from build123d import *

# Parameters (mm, degrees)
SKETCH2_W           = 10.16
SKETCH2_H           = 76.2
SKETCH2_W_2         = 50
SKETCH2_H_2         = 10.16
SKETCH2_H_3         = 89.916
SKETCH2_R           = 3.175
SKETCH2_H_4         = 10
SKETCH2_R_2         = 4.7625
BOSS_EXTRUDE1_DEPTH = 10.16
SKETCH6_W           = 14
SKETCH6_H           = 112.399749
CUT_EXTRUDE1_DEPTH  = 15.24
CUT_EXTRUDE2_START  = -10.16
SKETCH11_R          = 4
CUT_EXTRUDE2_DEPTH  = 10.16


with BuildPart() as part:
    # Sketch2 → Boss-Extrude1 (new body)
    with BuildSketch(Plane.XY):
        with BuildLine():
            Line((-408.300796745, 142.616356263), (-408.921789204, 152.75736057))
            Line((-408.921789204, 152.75736057), (-459.721789204, 152.75736057))
            Line((-459.721789204, 152.75736057), (-459.721789204, 76.39736057))
            Line((-459.721789204, 76.39736057), (-469.435656714, 76.39736057))
            Line((-469.435656714, 76.39736057), (-469.435656714, 25.59736057))
            Line((-469.435656714, 25.59736057), (-459.721789204, 25.59736057))
            Line((-459.721789204, 25.59736057), (-459.721789204, -230.782639429))
            ThreePointArc((-459.721789204, -230.782639429), (-437.403325931, -284.664176156), (-383.521789204, -306.982639429))
            Line((-383.521789204, -306.982639429), (-303.52, -306.982639429))
            Line((-303.52, -306.982639429), (-270.8, -306.98263943))
            Line((-270.8, -306.98263943), (-270.8, -317.14263943))
            Line((-270.8, -317.14263943), (-220, -317.14263943))
            Line((-220, -317.14263943), (-220, -306.98263943))
            Line((-220, -306.98263943), (-55.8292, -306.982639429))
            Line((-55.8292, -306.982639429), (-55.8292, -317.14263943))
            Line((-55.8292, -317.14263943), (55.8292, -317.14263943))
            Line((55.8292, -317.14263943), (55.8292, -306.982639429))
            Line((55.8292, -306.982639429), (220, -306.98263943))
            Line((220, -306.98263943), (220, -317.14263943))
            Line((220, -317.14263943), (270.8, -317.14263943))
            Line((270.8, -317.14263943), (270.8, -306.98263943))
            Line((270.8, -306.98263943), (303.52, -306.982639429))
            Line((303.52, -306.982639429), (383.521789204, -306.982639429))
            ThreePointArc((383.521789204, -306.982639429), (437.403325931, -284.664176156), (459.721789204, -230.782639429))
            Line((459.721789204, -230.782639429), (459.721789204, 25.59736057))
            Line((459.721789204, 25.59736057), (469.435656714, 25.59736057))
            Line((469.435656714, 25.59736057), (469.435656714, 76.39736057))
            Line((469.435656714, 76.39736057), (459.721789204, 76.39736057))
            Line((459.721789204, 76.39736057), (459.721789204, 152.75736057))
            Line((459.721789204, 152.75736057), (408.921789204, 152.75736057))
            Line((408.921789204, 152.75736057), (408.921789204, 142.616356263))
            Line((408.921789204, 142.616356263), (332.721789204, 142.616356263))
            Line((332.721789204, 142.616356263), (332.721789204, 152.75736057))
            Line((332.721789204, 152.75736057), (84.450547773, 152.75736057))
            Line((84.450547773, 152.75736057), (84.450547773, 316.728644457))
            Line((84.450547773, 316.728644457), (-84.450547773, 316.728644457))
            Line((-84.450547773, 316.728644457), (-84.450547773, 152.75736057))
            Line((-84.450547773, 152.75736057), (-332.100796745, 152.75736057))
            Line((-332.100796745, 152.75736057), (-332.100796745, 142.616356263))
            Line((-332.100796745, 142.616356263), (-408.300796745, 142.616356263))
        make_face()
        with Locations((-205.08, -256.782661115)):
            Rectangle(SKETCH2_W, SKETCH2_H, mode=Mode.SUBTRACT)
        with Locations((-84.92, -256.782661115)):
            Rectangle(SKETCH2_W, SKETCH2_H, mode=Mode.SUBTRACT)
        with Locations((-345.16, -186.334154613)):
            Rectangle(SKETCH2_W_2, SKETCH2_H_2, mode=Mode.SUBTRACT)
        with Locations((-310.712287657, -172.10863943)):
            Rectangle(SKETCH2_W, SKETCH2_H_3, mode=Mode.SUBTRACT)
        with Locations((-436.123522935, -86.033983844)):
            Circle(SKETCH2_R, mode=Mode.SUBTRACT)
        with Locations((-405.323522935, -86.033983844)):
            Circle(SKETCH2_R, mode=Mode.SUBTRACT)
        with Locations((-235.16, -186.254154613)):
            Rectangle(SKETCH2_W_2, SKETCH2_H_4, mode=Mode.SUBTRACT)
        with Locations((310.712287657, -172.10863943)):
            Rectangle(SKETCH2_W, SKETCH2_H_3, mode=Mode.SUBTRACT)
        with Locations((-345.16, -74.366988355)):
            Rectangle(SKETCH2_W_2, SKETCH2_H_2, mode=Mode.SUBTRACT)
        with Locations((-310.712287657, 7.72336057)):
            Rectangle(SKETCH2_W, SKETCH2_H_3, mode=Mode.SUBTRACT)
        Polygon((-210.16, -79.446988355), (-260.16, -79.446988355), (-260.16, -69.446988355), (-210.16, -69.446988355), (-210.16, -8.96237531), (-200, -8.96237531), (-200, -85.16237531), (-210.16, -85.16237531), align=None, mode=Mode.SUBTRACT)
        with Locations((-84.92, -47.06237531)):
            Rectangle(SKETCH2_W, SKETCH2_H, mode=Mode.SUBTRACT)
        with Locations((-436.123522935, 60.016016156)):
            Circle(SKETCH2_R, mode=Mode.SUBTRACT)
        with Locations((-405.323522935, 60.016016156)):
            Circle(SKETCH2_R, mode=Mode.SUBTRACT)
        with Locations((-420.723522935, 122.038203417)):
            Circle(SKETCH2_R, mode=Mode.SUBTRACT)
        with Locations((-172.2755, 25.75736057)):
            Circle(SKETCH2_R_2, mode=Mode.SUBTRACT)
        with Locations((-81.7245, 25.75736057)):
            Circle(SKETCH2_R_2, mode=Mode.SUBTRACT)
        with Locations((-172.2755, 127.35736057)):
            Circle(SKETCH2_R_2, mode=Mode.SUBTRACT)
        with Locations((-81.7245, 127.35736057)):
            Circle(SKETCH2_R_2, mode=Mode.SUBTRACT)
        with Locations((310.712287657, 7.72336057)):
            Rectangle(SKETCH2_W, SKETCH2_H_3, mode=Mode.SUBTRACT)
        with Locations((81.7245, 25.75736057)):
            Circle(SKETCH2_R_2, mode=Mode.SUBTRACT)
        with Locations((81.7245, 127.35736057)):
            Circle(SKETCH2_R_2, mode=Mode.SUBTRACT)
        with Locations((172.2755, 25.75736057)):
            Circle(SKETCH2_R_2, mode=Mode.SUBTRACT)
        with Locations((172.2755, 127.35736057)):
            Circle(SKETCH2_R_2, mode=Mode.SUBTRACT)
    extrude(amount=-BOSS_EXTRUDE1_DEPTH)

    # Sketch6 → Cut-Extrude1 (cut)
    with BuildSketch(Plane(origin=(0, 0, -10.16), x_dir=(-1, 0, 0), z_dir=(0, 0, -1))):
        with Locations((386.721789204, 30.216607763)):
            Rectangle(SKETCH6_W, SKETCH6_H)
        with Locations((386.721789204, -194.582890237)):
            Rectangle(SKETCH6_W, SKETCH6_H)
    cut_extrude1 = extrude(amount=-CUT_EXTRUDE1_DEPTH, mode=Mode.SUBTRACT)

    # Mirror1: Cut-Extrude1 across plane
    add(cut_extrude1.mirror(Plane(origin=(0, 0, 0), x_dir=(0, 0, 1), z_dir=(1, 0, 0))), mode=Mode.SUBTRACT)

    # Sketch11 → Cut-Extrude2 (cut)
    with BuildSketch(Plane.XY.offset(CUT_EXTRUDE2_START)):
        with Locations((-172.6526, -269.442639029)):
            Circle(SKETCH11_R)
        with BuildLine():
            Line((-168.652969828, -239.497030969), (-176.652230173, -239.497030969))
            ThreePointArc((-176.652230173, -239.497030969), (-172.6526, -243.442639029), (-168.652969828, -239.497030969))
        make_face()
        with BuildLine():
            ThreePointArc((-168.6526, -239.442639029), (-172.679796599, -235.442731487), (-176.652230173, -239.497030969))
            Line((-176.652230173, -239.497030969), (-168.652969828, -239.497030969))
            ThreePointArc((-168.652969828, -239.497030969), (-168.652692458, -239.469835628), (-168.6526, -239.442639029))
        make_face()
        with BuildLine():
            ThreePointArc((-113.3474, -239.442639029), (-117.374596599, -235.442731487), (-121.347030173, -239.497030969))
            Line((-121.347030173, -239.497030969), (-113.347769828, -239.497030969))
            ThreePointArc((-113.347769828, -239.497030969), (-113.347492458, -239.469835628), (-113.3474, -239.442639029))
        make_face()
        with BuildLine():
            Line((-113.347769828, -239.497030969), (-121.347030173, -239.497030969))
            ThreePointArc((-121.347030173, -239.497030969), (-117.3474, -243.442639029), (-113.347769828, -239.497030969))
        make_face()
        with Locations((-117.3474, -269.442639029)):
            Circle(SKETCH11_R)
    extrude(amount=CUT_EXTRUDE2_DEPTH, mode=Mode.SUBTRACT)


solid = part.part
Input: part model. Units: mm. Frame: model coordinates. Coordinates: 2 decimals unless noted, no trailing zeros. Loops run counter-clockwise (first coordinate to the right, second up) from the corner with the lowest first, then second, coordinate; pieces in that order, holes last. Notation, with made-up numbers: (33.5, 30) -> (58.5, 30) arc R27 cw to (58.5, 46) -> close; hole circle Ø1 at (-32, 8.5). An arc over 180 degrees is marked (long way). Write item = value, one per line. Start each with the question number.
Item 1: Cut plane D-D, the plane y = 194. Return loops of the section in (x, z), plus the area to 3 significant figures.
Item 2: Mould query, pull axis Z, two halves, no side actions, for faces 1 (the face through (-7, -66, -10.16)), 2 (the face through (-7, -66, 0)), 3 (the face through (-437.99, -284.07, -5.01)). Classes: pulls with the +Z half, pulls with the -Z half, needs draft (parallel to the pull), parting line crosses it, or undercut.
Item 3: Cut plane C-C, the plane z = -6.75. Count the separate pieces of the cut face and the enclosed holes in it, plus the area to 3 significant figures.
Item 4: First-contact query: P1, Ø3, axis at y = -83.5, z = -4.5, coming from the +X side; P2, Ø3, axis at y = -243.5, z = -3.5, coming from the +X side; P3, Ø3, axis at x = 388.5, z = -3, coming from the -Y side. Flat tips, straight axial feed; report the tip coordinate or a pass-through.
Item 5: Cut plane A-A, the plane x = -343.5. Return loops of the section in (y, z), plus the area to 3 significant figures.
Item 6: Cut plane B-B, the plane x = 127.5. Return loops of the section in (y, z).
Item 7: Material intervals for line 1 (Y direction, x = -172.5, z = -0.75); line 2 (X direction, y = -132.5, z = -8); line 3 (X direction, y = -6, z = -4), sorted ascending.
Ans:
q1.outline = (-84.45, -10.16) -> (84.45, -10.16) -> (84.45, 0) -> (-84.45, 0) -> close
q1.area = 1,720 mm²
q2.face_1 = pulls with the -Z half
q2.face_2 = pulls with the +Z half
q2.face_3 = needs draft
q3.separate_pieces = 1
q3.enclosed_holes = 32
q3.area = 434,000 mm²
q4.P1 = 459.72
q4.P2 = 458.89
q4.P3 = -306.9
q5.outline = (-306.98, -10.16) -> (-191.41, -10.16) -> (-191.41, 0) -> (-306.98, 0) -> close; (-181.25, -10.16) -> (-79.45, -10.16) -> (-79.45, 0) -> (-181.25, 0) -> close; (-69.29, -10.16) -> (142.62, -10.16) -> (142.62, 0) -> (-69.29, 0) -> close
q5.area = 4,360 mm²
q6.outline = (-306.98, -10.16) -> (152.76, -10.16) -> (152.76, 0) -> (-306.98, 0) -> close
q7.line_1 = -306.98 to -273.44, -265.45 to -243.44, -235.45 to 21, 30.51 to 122.6, 132.11 to 152.76
q7.line_2 = -459.72 to -315.79, -305.63 to 305.63, 315.79 to 459.72
q7.line_3 = -459.72 to -393.72, -379.72 to -315.79, -305.63 to 305.63, 315.79 to 379.72, 393.72 to 459.72
